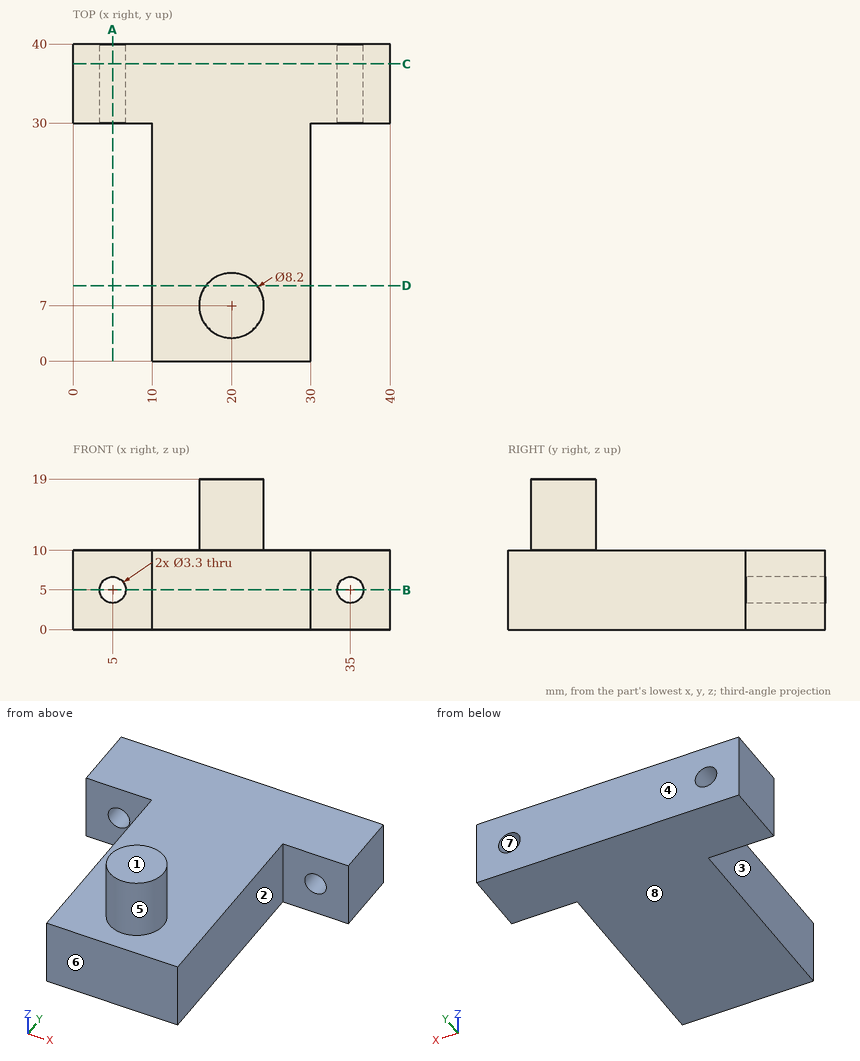
Answer from the drawing. Dimensions are ordinates in mm from the lowest x, y and z of the part. A direction names the side the tool comes from. Round coordinates to 2 decimals unless told otherwise and drop trailing zeros. Write each loop counter-clockwise with the first axis right and the second up, starting at its lowest first coordinate (ties: lowest second). Pieces come first, ordered by that corner, then holes.
1. Determine the mould class of the marked faces 6, 7 and 8 for opening direction Z: pulls with the +Z half, pulls with the -Z half, needs draft (parallel to the pull), parting line crosses it, or undercut.
2. The part is cut by section D-D, the plane y = 9.5. Determine the outline of the cut face in (x, z), then the cut area to 3 significant figures.
3. The part is cut by section A-A, the plane x = 5. Determine the outline of the cut face in (y, z).
4. Straight lines are drawn through the part: L1, parallel to X at y = 37.5, z = 5; L2, parallel to Z at x = 35, y = 35; L3, parallel to Y at x = 32, z = 1. For each, find the intervals that lie inside material, in ascending order.
5. Which of the six approach directions +Z, -Z, +X, -X, +Y, -Y give full straight-line access (tool end or side, diameter ignored) to the marked faces 1, 2, 3, 4 and 5?
6. Given pin 1 Ø3 at (y, z) = (11.5, 5.5) entering from +X; pin 2 Ø5 at (y, z) = (8, 3.5) entering from -X; pin 3 Ø5.5 at (x, z) = (5, 5) entering from -Y, each flat-ended and moving along its own axis, determine where each tip first touches the part or whether it passes through.
7. The part is cut by section C-C, the plane y = 37.5. Determine the outline of the cut face in (x, z).
8. The part is cut by section B-B, the plane z = 5. Determine the outline of the cut face in (x, y).
Values:
1. face 6: needs draft
1. face 7: undercut
1. face 8: pulls with the -Z half
2. outline: (10, 0) - (30, 0) - (30, 10) - (23.25, 10) - (23.25, 19) - (16.75, 19) - (16.75, 10) - (10, 10) - close
2. area: 258 mm2
3. outline: (30, 0) - (40, 0) - (40, 3.35) - (30, 3.35) - close; (30, 6.65) - (40, 6.65) - (40, 10) - (30, 10) - close
4. L1: x = 0 to 3.35, 6.65 to 33.35, 36.65 to 40
4. L2: z = 0 to 3.35, 6.65 to 10
4. L3: y = 30 to 40
5. face 1: +Z, +X, -X, +Y, -Y
5. face 2: +Z, -Z, +X, -Y
5. face 3: +Z, -Z, -X, -Y
5. face 4: +Z, -Z, +X, -X, +Y
5. face 5: +Z
6. pin 1: stops at x = 30
6. pin 2: stops at x = 10
6. pin 3: stops at y = 30
7. outline: (0, 0) - (40, 0) - (40, 10) - (0, 10) - close; hole circle Ø3.3 at (5, 5); hole circle Ø3.3 at (35, 5)
8. outline: (0, 30) - (3.35, 30) - (3.35, 40) - (0, 40) - close; (6.65, 30) - (10, 30) - (10, 0) - (30, 0) - (30, 30) - (33.35, 30) - (33.35, 40) - (6.65, 40) - close; (36.65, 30) - (40, 30) - (40, 40) - (36.65, 40) - close
